Input: part model. Units: mm. Frame: model coordinates. A direction names the side the tool comes from. Give positions to 0.01 mm unless a question says otherwise; leave off trailing zeros. Loops run counter-clockwise (first coordinate to the right, second up) from the corner with the lowest first, then second, coordinate; pieces in that order, holes last. Notation, with made-up numbers: (59.5, 6.5) -> (84.5, 6.5) arc R26 cw to (84.5, 34.5) -> close; hole circle Ø2 at (45.5, -30). An arc over 180 degrees is marked (long way). Use CSV: the item, a comma, the result in double quotes.
```python
from build123d import *

# Parameters (mm, degrees)
CHAMFER1_SIZE     = 0.635
CIRPATTERN1_COUNT = 3
FILLET1_R         = 0.9652


with BuildPart() as part:
    # Sketch1 → Revolve1 (revolve)
    with BuildSketch(Plane.XY, mode=Mode.PRIVATE) as revolve1_sk:
        Polygon((0, 0), (0, 7.9375), (1.984375, 7.9375), (1.984375, 3.175), (52.784375, 3.175), (52.784375, 0), align=None)
    revolve(revolve1_sk.sketch.rotate(Axis((0, 0, 0), (1, 0, 0)), 180), axis=Axis((0, 0, 0), (1, 0, 0)))

    # Chamfer1
    chamfer1_edges = [part.edges().sort_by_distance(p)[0] for p in [
        (52.784375, 3.175, 0),
    ]]
    chamfer(chamfer1_edges, length=CHAMFER1_SIZE)

    # Sketch2 → Revolve2 (revolve)
    with BuildSketch(Plane.XY, mode=Mode.PRIVATE) as revolve2_sk:
        with BuildLine():
            Line((1.984375, -5.55625), (2.949575, -5.55625))
            ThreePointArc((2.949575, -5.55625), (2.678583674, -4.783713061), (1.984375, -4.34975))
            Line((1.984375, -4.34975), (1.984375, -5.55625))
        make_face()
    revolve2 = revolve(revolve2_sk.sketch.rotate(Axis((1.984375, -5.55625, 0), (-1, 0, 0)), 180), axis=Axis((1.984375, -5.55625, 0), (-1, 0, 0)))

    # CirPattern1: Revolve2 ×3 about axis
    cirpattern1_axis = Axis((0, 0, 0), (1, 0, 0))
    for i in range(1, CIRPATTERN1_COUNT):
        add(revolve2.rotate(cirpattern1_axis, i * 360 / CIRPATTERN1_COUNT))

    # Fillet1
    fillet1_edges = [part.edges().sort_by_distance(p)[0] for p in [
        (1.984375, 3.175, 0),
        (0, 7.9375, 0),
    ]]
    fillet(fillet1_edges, radius=FILLET1_R)


solid = part.part
```
1) Ray query, line 1 (X direction, y = 4, z = 0.5); line 2 (Z direction, x = 39.5, y = 2.75); line 3 (Z direction, x = 19.5, y = 2.5). Return the intervals inside material, ascending.
From the geometry:
line 1,"x = 0 to 1.99"
line 2,"z = -1.59 to 1.59"
line 3,"z = -1.96 to 1.96"
2) Section query A-A (y = 0). Return loops of the section in (x, z) (1 decimal), then the cut area to 3 significant figures.
From the geometry:
outline,"(0, -7) arc R1 ccw to (1, -7.9) -> (2, -7.9) -> (2, -4.1) arc R1 cw to (2.9, -3.2) -> (52.1, -3.2) -> (52.8, -2.5) -> (52.8, 2.5) -> (52.1, 3.2) -> (2.9, 3.2) arc R1 cw to (2, 4.1) -> (2, 7.9) -> (1, 7.9) arc R1 ccw to (0, 7) -> close"
area,"354 mm^2"
3) Contact query for flat-ended pins moving along their axis: pin 1 (2 mm diameter, centred on y = -3, z = -5, fed in from +X); pin 2 (3 mm diameter, centred on x = 15, z = -3.5, fed in from +Y); pin 3 (8 mm diameter, centred on x = 14, z = -5, fed in from -Y); pin 4 (4 mm diameter, centred on y = 2.5, z = 1.5, fed in from +X). Output: stop coordinate, or through.
From the geometry:
pin 1,"stops at x = 1.98"
pin 2,"stops at y = 2.47"
pin 3,"stops at y = -3.01"
pin 4,"stops at x = 52.78"
4) Section query C-C (x = 15). Return loops of the section in (y, z) (3 decimals), then the cut area to 3 significant figures.
From the geometry:
outline,"circle Ø6.35 at (0, 0)"
area,"31.7 mm^2"
5) Reachability of faces 1 (the flat face through (52.784, 0, 0)), 2 (the flat face through (1.984, -3.4, 3.4)) from +Z, -Z, +X, -X, +Y, -Y: full face, straight path, thin tool, end or side. Return the list, or none.
From the geometry:
face 1,"+Z, -Z, +X, +Y, -Y"
face 2,"+X"
